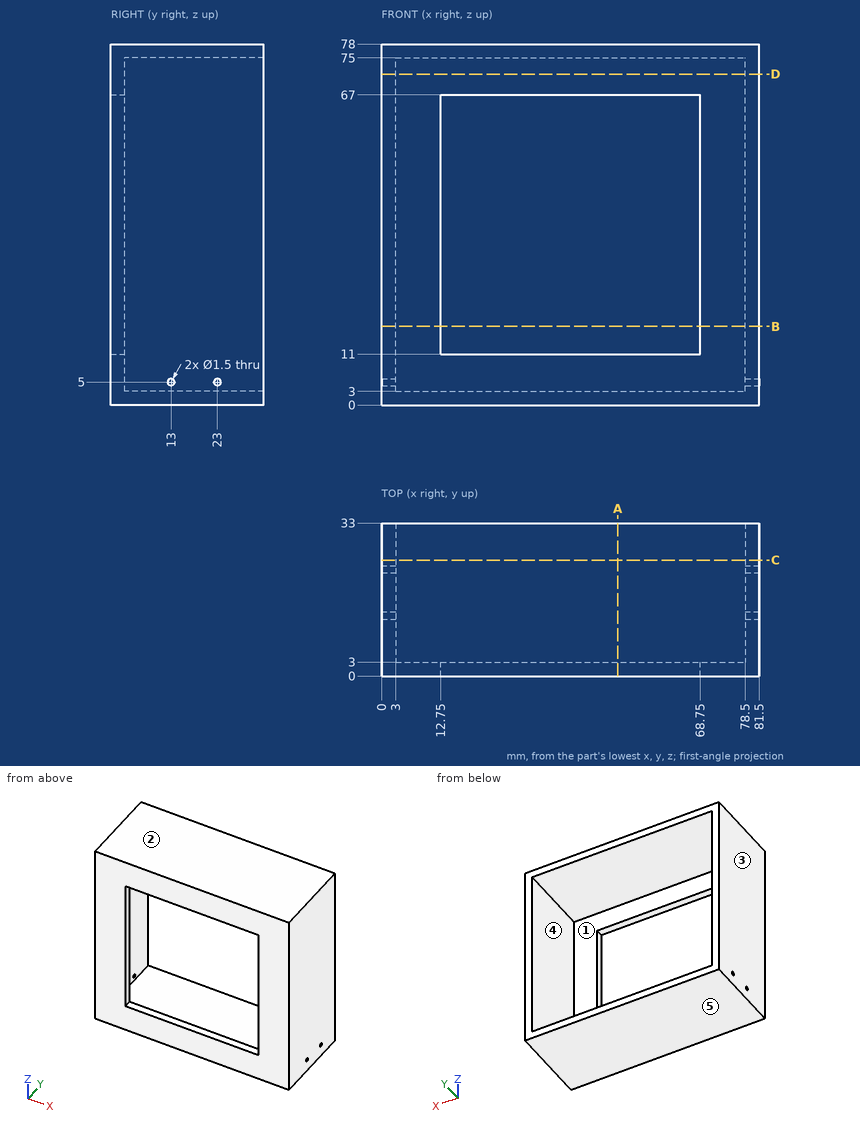
Geometry check sheet. Reference: drawing and pictorial views, mm from the part's lowest x, y, z. A direction names the side the tool comes from. Give positions to 0.01 mm unless a question says otherwise; leave off trailing zeros. Order: outer loops, then holes, each group sorted by start corner. A loop starts at its lowest first (then second) coordinate and runs counter-clockwise, first axis right, second up. Notation, with made-up numbers: M -4.75,21 L 31.25,21 A26 cw 31.25,44 Z; hole C 69,80 d4. An arc over 180 degrees is marked long. Answer in a Markdown table with one row per item. Add a question column.
Item 1: Section check A-A, the plane x = 51. Enter the section's corners in (y, z).
Item 2: Mould release check, pull along X, two halves, no side actions. Record for the marked faces 1, 2 and 3: released by +X, released by -X, zero draft, split by the parting line, or undercut.
Item 3: Scan lines: probe 1 along X at (y, z) = (18, 69.5); probe 2 along Z at (x, y) = (79.5, 23); probe 3 along Z at (x, y) = (7, 5). Record each from-to range of solid material in increasing order. Write a range as from..to.
Item 4: Section check D-D, the plane z = 71.5. Enter the section's corners in (x, y), and give its area (4 significant figures).
Item 5: Tool access check on the marked faces 4 and 5. Record the directions out of +Z, -Z, +X, -X, +Y, -Y that give a thin tool (end or side, any length) a straight path to the whole face; none if there is none.
Item 6: Section check C-C, the plane y = 25. Enter the section's corners in (x, z), and give its area (3 significant figures).
Item 7: Section check B-B, the plane z = 17. Enter the section's corners in (x, y).
Item 8: Gauge pin test, flat end, axial feed: pin 1 (10 mm diameter, centred on x = 18.5, z = 9.5, fed in from +Y). Record the tip position at first contact, or that the pin passes through.
Filled sheet:
| question | item | result |
|---|---|---|
| 1 | outline | M 0,0 L 33,0 L 33,3 L 3,3 L 3,11 L 0,11 Z; M 0,67 L 3,67 L 3,75 L 33,75 L 33,78 L 0,78 Z |
| 2 | face 1 | undercut |
| 2 | face 2 | zero draft |
| 2 | face 3 | released by -X |
| 3 | probe 1 | x = 0..3, 78.5..81.5 |
| 3 | probe 2 | z = 0..4.25, 5.75..78 |
| 3 | probe 3 | z = 0..3, 75..78 |
| 4 | outline | M 0,0 L 81.5,0 L 81.5,33 L 78.5,33 L 78.5,3 L 3,3 L 3,33 L 0,33 Z |
| 4 | area | 424.5 mm^2 |
| 5 | face 4 | +Y |
| 5 | face 5 | -Z, +X, -X, +Y, -Y |
| 6 | outline | M 0,0 L 81.5,0 L 81.5,78 L 0,78 Z; hole M 3,3 L 78.5,3 L 78.5,75 L 3,75 Z |
| 6 | area | 921 mm^2 |
| 7 | outline | M 0,0 L 12.75,0 L 12.75,3 L 3,3 L 3,33 L 0,33 Z; M 68.75,0 L 81.5,0 L 81.5,33 L 78.5,33 L 78.5,3 L 68.75,3 Z |
| 8 | pin 1 | stops at y = 3 |
